Autodesk Inventor part; units mm, degrees
ref_plane "YZ Plane" through (0, 0, 0) normal (1, 0, 0) x (0, 1, 0)
ref_plane "XZ Plane" through (0, 0, 0) normal (0, 1, 0) x (-1, 0, 0)
ref_plane "XY Plane" through (0, 0, 0) normal (0, 0, 1) x (1, 0, 0)
sketch "Szkic2" plane through (0, 0, 0) normal (0, 1, 0) x (-1, 0, 0)
  line L0 (42.5, 23) -> (-42.5, 23)
  line L1 (-42.5, 23) -> (-42.5, -23)
  line L2 (-42.5, -23) -> (42.5, -23)
  line L3 (42.5, -23) -> (42.5, 23)
  line L4 (0, 91.0722) -> (0, -100.1143)
  line L5 (-78.4738, 0) -> (170.7955, 0)
  circle A0 centre (37.932, 17.8265) radius 2
  circle A1 centre (37.932, -17.8265) radius 2
  circle A2 centre (-37.932, 17.8265) radius 2
  circle A3 centre (-37.932, -17.8265) radius 2
  point P0 (0, 0)
  dimension "d7" = 46
  dimension "d8" = 85
  dimension "d14" = 4
  dimension "d16" = 35.653
  dimension "d18" = 23
  dimension "d21" = 75.864
  dimension "d22" = 42.5
extrude "Wyciągnięcie proste2" add sketch "Szkic2" along normal blind 2
sketch "Szkic3" plane through (0, 2, 0) normal (0, 1, 0) x (1, 0, 0)
  line L0 (-42.5, -23) -> (42.5, -23)
  line L1 (42.5, -23) -> (42.5, 23)
  line L2 (41.3, -23) -> (42.5, -23)
  line L3 (42.5, -23) -> (42.5, 23)
  line L4 (42.5, 23) -> (41.3, 23)
  line L5 (41.3, 23) -> (41.3, -23)
  line L6 (-42.5, 23) -> (-42.5, -23)
  line L7 (42.5, -23) -> (-42.5, -23)
  line L8 (-42.5, -23) -> (-42.5, -21.8)
  line L9 (-42.5, -21.8) -> (42.5, -21.8)
  line L10 (42.5, -21.8) -> (42.5, -23)
  line L11 (42.5, 23) -> (-42.5, 23)
  line L12 (-42.5, 23) -> (-42.5, 21.8)
  line L13 (-42.5, 21.8) -> (42.5, 21.8)
  line L14 (42.5, 21.8) -> (42.5, 23)
  line L15 (42.5, 23) -> (-42.5, 23)
  line L16 (-42.5, -23) -> (-41.3, -23)
  line L17 (-41.3, -23) -> (-41.3, 23)
  line L18 (-41.3, 23) -> (-42.5, 23)
  line L19 (-42.5, 23) -> (-42.5, -23)
  line L20 (42.5, -6) -> (41.3, -6)
  line L21 (41.3, -6) -> (41.3, 6)
  line L22 (41.3, 6) -> (42.5, 6)
  line L23 (36.3786, 0) -> (45.7918, 0)
  point P0 (0, 0)
  point P1 (41.3, -21.8)
  point P2 (-41.3, -21.8)
  point P3 (-41.3, 21.8)
  point P4 (41.3, 21.8)
  dimension "d25" = 1.2
  dimension "d26" = 1.2
  dimension "d27" = 1.2
  dimension "d28" = 1.2
  dimension "d29" = 12
  dimension "d30" = 6
extrude "Wyciągnięcie proste3" add sketch "Szkic3" along normal blind 10 contours L6 L9 L17 L0 | L17 L9 L5 L0 | L6 L13 L17 L9 | L5 L9 L1 L0 | L6 L11 L17 L13 | L5 L20 L1 L9 | L17 L11 L5 L13 | L13 L1 L22 L5 | L5 L4 L1 L13
sketch "Szkic5" plane through (0, 12, 0) normal (0, 1, 0) x (1, 0, 0)
  line L0 (41.3, -6) -> (41.3, -21.8)
  line L1 (42.5, -6) -> (42.5, 6)
  line L2 (41.3, -8) -> (42.5, -8)
  line L3 (42.5, -8) -> (42.5, -2)
  line L4 (42.5, -2) -> (41.3, -2)
  line L5 (41.3, -2) -> (41.3, -8)
  line L6 (34.6755, 0) -> (49.4443, 0)
  line L7 (40.0187, -6) -> (43.7777, -6)
  line L8 (41.3, 8) -> (42.5, 8)
  line L9 (42.5, 8) -> (42.5, 2)
  line L10 (42.5, 2) -> (41.3, 2)
  line L11 (41.3, 2) -> (41.3, 8)
  line L12 (40.0187, 6) -> (43.7777, 6)
  point P0 (0, 0)
  point P1 (41.3, 6)
  dimension "d33" = 6
  dimension "d34" = 2
extrude "Wyciągnięcie proste4" add sketch "Szkic5" along normal blind 1 contours L7 L3 L2 L0 | L12 L11 L8 L9
extrude "Wyciągnięcie proste5" add sketch "Szkic5" along normal mid plane 2 contours L10 L11 L12 L1 | L5 L4 L1 L7
sketch "Szkic6" plane through (42.5, 0, -23) normal (0, 0, -1) x (-1, 0, 0)
  line L0 (83.8, 12) -> (1.2, 12)
  line L1 (26, 12) -> (26, 0)
  line L2 (31.5, 12) -> (31.5, 0)
  line L3 (53.5, 12) -> (53.5, 0)
  line L4 (0, 0) -> (85, 0)
  line L5 (56.5, 12) -> (56.5, 0)
  line L6 (0, 0) -> (0, 12)
  circle A0 centre (28.6456, 7.207) radius 1.5875
  line L7 (1.2, 2) -> (83.8, 2)
  line L8 (26, 2) -> (56.5, 2)
  point P0 (42.5, 0)
  dimension "d39" = 5.5
  dimension "d40" = 22
  dimension "d41" = 3
  dimension "d42" = 31.5
  dimension "d43" = 3.175
  dimension "d55" = 5.207
sketch "Szkic8" plane through (0, 0, 0) normal (0, -1, 0) x (1, 0, 0)
  line L0 (42.5, -23) -> (-42.5, -23)
  line L1 (20.6822, -23) -> (-15.9857, -23)
  line L2 (-15.9857, -23) -> (-15.9857, -42.1071)
  line L3 (-15.9857, -42.1071) -> (20.6822, -42.1071)
  line L4 (20.6822, -42.1071) -> (20.6822, -23)
  line L5 (17, -23) -> (11, -23)
  line L6 (11, -23) -> (11, -35.8)
  line L7 (11, -35.8) -> (17, -35.8)
  line L8 (17, -35.8) -> (17, -23)
  line L9 (11, -23) -> (-11, -23)
  line L10 (-11, -23) -> (-11, -35.8)
  line L11 (-11, -35.8) -> (11, -35.8)
  line L12 (11, -35.8) -> (11, -23)
  line L13 (-11, -23) -> (-14, -23)
  line L14 (-14, -23) -> (-14, -35.8)
  line L15 (-14, -35.8) -> (-11, -35.8)
  line L16 (-11, -35.8) -> (-11, -23)
  line L17 (17, -26.8) -> (-14, -26.8)
  point P0 (0, 0)
  point P1 (11, -26.8)
  point P2 (-14, -23)
  point P3 (17, -23)
  dimension "d45" = 6
  dimension "d46" = 22
  dimension "d47" = 3
  dimension "d48" = 31.5
  dimension "d49" = 3.8
  dimension "d50" = 9
extrude "Wyciągnięcie proste6" add sketch "Szkic8" against normal blind 2 contours L6 L17 L10 L0 | L8 L7 L6 L17 | L10 L17 L14 L0 | L6 L11 L10 L17 | L10 L15 L14 L17
extrude "Wyciągnięcie proste7" add sketch "Szkic8" against normal blind 12 contours L8 L17 L6 L0
sketch "Szkic9" plane through (17, 2, -26.8) normal (0, 0, -1) x (-1, 0, 0)
  circle A0 centre (3.0287, 5.207) radius 1.4322
  line L0 (0, 0) -> (31, 0)
  point P0 (17, -2)
  dimension "d63" = 5.207
hole "Otwór2" at (13.9713, 7.207, -26.8) direction (0, 0, 1) diameter 4 depth 4 counterbore diameter 4.5 counterbore depth 0.6
properties part number "prent1"
Design review of the part built by this model. Coordinates are the model's own, in mm. A direction names the side the tool comes from. Give positions to 0.01 mm unless a question says otherwise; leave off trailing zeros. Order: outer loops, then holes, each group sorted by start corner. A loop starts at its lowest first (then second) coordinate and runs counter-clockwise, first axis right, second up. Notation, with made-up numbers: M -26,76.25 L 7,76.25 A19 cw 7,102.25 Z; hole C 18.25,-39.5 d3. An arc over 180 degrees is marked long. One line per question, with ' | ' between items. Start each with the question number.
Q1. We need section A-A (x = -37). Write out the cut boundary in (y, z), plus the area to 3 significant figures.
Q2. We need section C-C (x = -3). Write out the cut boundary in (y, z).
Q3. For L1, parallel to X at y = 2.5, z = 8; L2, parallel to Z at x = -13, y = 5.25; L3, parallel to Y at x = 15, z = -2.5, list the stretches that pass through material, from the lowest coordinate up. Write a range as [from, to].
Q4. The part is to be moulded in two halves that separate along X. For faces 1 (the face through (11, 7, -25)), 2 (the face through (-1, 7, -21.8)), 3 (the face through (36.085, 0.986, -17.06)), 4 (the face through (1, 1, -35.8)), say which applies: +X half, -X half, draft (parallel to the pull), parting line (faces both ways), or undercut.
Q5. We need section B-B (z = -10). Write out the cut boundary in (x, y), plus the area to 3 significant figures.
Q6. For pin 1 Ø3.5 at (x, z) = (37.93, -17.83) entering from +Y; pin 2 Ø4.5 at (x, z) = (-37.93, -17.83) entering from +Y; pin 3 Ø0.5 at (x, y) = (42, 12.5) entering from -Z; pin 4 Ø0.6 at (x, y) = (41.5, 5) entering from -Z, all flat-tipped, find the tip position at first contact; note any pin that passes through.
Q7. Machinability: for faces 5 (the face through (13.371, 9.115, -24.476)), 6 (the face through (14, 4.7, -26.8)), 7 (the face through (-41.3, 7, 0)), 8 (the face through (17, 4.6, -26.6)), 9 (the face through (-1, 0, 1)), which of the approach directions +Z, -Z, +X, -X, +Y, -Y give a long, thin tool a straight path to every point of the face, cutting with its end or side? Answer none if there is none.
Q8. We need section D-D (z = 7). Write out the cut boundary in (x, y).
Returned:
1) outline: M 0,-23 L 12,-23 L 12,-21.8 L 2,-21.8 L 2,-19.6 L 0,-19.6 Z; M 0,-16.06 L 2,-16.06 L 2,16.06 L 0,16.06 Z; M 0,19.6 L 2,19.6 L 2,21.8 L 12,21.8 L 12,23 L 0,23 Z | area: 102 mm2
2) outline: M 0,-35.8 L 2,-35.8 L 2,-23 L 12,-23 L 12,-21.8 L 2,-21.8 L 2,21.8 L 12,21.8 L 12,23 L 0,23 Z
3) L1: [-42.5, -41.3], [41.3, 42.5] | L2: [-23, -21.8], [21.8, 23] | L3: [0, 2]
4) face 1: -X half | face 2: undercut | face 3: undercut | face 4: draft
5) outline: M -42.5,0 L 42.5,0 L 42.5,12 L 41.3,12 L 41.3,2 L -41.3,2 L -41.3,12 L -42.5,12 Z | area: 194 mm2
6) pin 1: through | pin 2: y = 2 | pin 3: z = -8 | pin 4: z = -23
7) face 5: -Z | face 6: -Z, +X, -X, +Y | face 7: +Y | face 8: -Z, +X, +Y, -Y | face 9: +Z, -Z, +X, -X, -Y
8) outline: M -42.5,0 L 42.5,0 L 42.5,13 L 41.3,13 L 41.3,2 L -41.3,2 L -41.3,12 L -42.5,12 Z
